```python
from build123d import *

# Parameters (mm, degrees)
SKETCH1_W           = 76.2
SKETCH1_H           = 25.4
SKETCH1_W_2         = 69.85
SKETCH1_H_2         = 19.05
BOSS_EXTRUDE1_DEPTH = 254
SKETCH2_R           = 3.3782
CUT_EXTRUDE1_DEPTH  = 26.4
SKETCH3_R           = 3
CUT_EXTRUDE2_DEPTH  = 26.4


with BuildPart() as part:
    # Sketch1 → Boss-Extrude1 (new body)
    with BuildSketch(Plane(origin=(0, 0, 0), x_dir=(1, 0, 0), z_dir=(0, 1, 0))):
        with Locations((38.1, 12.7)):
            Rectangle(SKETCH1_W, SKETCH1_H)
        with Locations((38.1, 12.7)):
            Rectangle(SKETCH1_W_2, SKETCH1_H_2, mode=Mode.SUBTRACT)
    extrude(amount=BOSS_EXTRUDE1_DEPTH)

    # Sketch2 → Cut-Extrude1 (cut, through all)
    with BuildSketch(Plane(origin=(0, 0, -25.4), x_dir=(-1, 0, 0), z_dir=(0, 0, -1))):
        with Locations((-60.325, 15.875)):
            Circle(SKETCH2_R)
        with Locations((-15.875, 15.875)):
            Circle(SKETCH2_R)
        with Locations((-15.875, 60.325)):
            Circle(SKETCH2_R)
        with Locations((-60.325, 60.325)):
            Circle(SKETCH2_R)
    extrude(amount=-CUT_EXTRUDE1_DEPTH, mode=Mode.SUBTRACT)

    # Sketch3 → Cut-Extrude2 (cut, through all)
    with BuildSketch(Plane(origin=(0, 0, -25.4), x_dir=(-1, 0, 0), z_dir=(0, 0, -1))):
        with Locations((-65.347432125, 185.7375)):
            Circle(SKETCH3_R)
        with Locations((-65.347432125, 233.3625)):
            Circle(SKETCH3_R)
    extrude(amount=-CUT_EXTRUDE2_DEPTH, mode=Mode.SUBTRACT)


solid = part.part
```
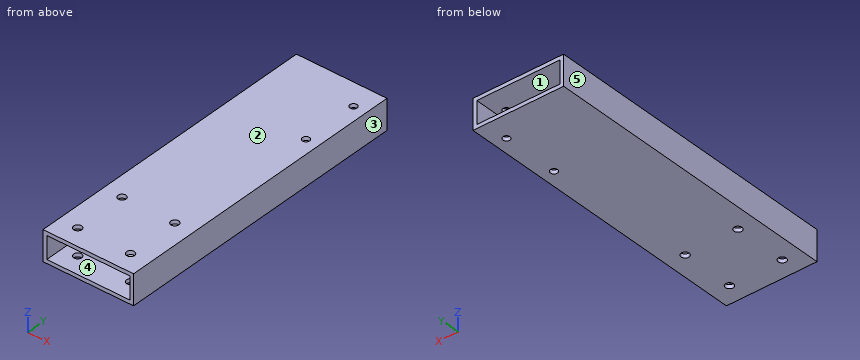
Could you check a few things on this model? Use its own coordinates, in mm. Face numbers are marked on the shaded views. A direction names the side the tool comes from. Coordinates: 2 decimals unless noted, no trailing zeros. Write each loop counter-clockwise with the first axis right and the second up, starting at its lowest first coordinate (ties: lowest second). Pieces come first, ordered by that corner, then holes. Notation, with made-up numbers: (58, 31) -> (94, 31) arc R23 cw to (94, 65) -> close; hole circle Ø3 at (-27, -3.75). An arc over 180 degrees is marked (long way). Return JSON: item names as keys, results as strings.
(1) I'm going to push a flat-ended pin straight in: pin 1 (4 mm diameter, centred on x = 15.875, y = 15.875, fed in from -Z). Where does the tip first touch, or does it pass through?
Numbers:
{"pin 1": "passes through"}
(2) Imagine slicing it at A-A, the plane x = 41. Please give me the cut outline in (y, z) (3 decimals), then the cut area to 3 significant figures.
Numbers:
{"outline": "(0, -25.4) -> (254, -25.4) -> (254, -22.225) -> (0, -22.225) -> close; (0, -3.175) -> (254, -3.175) -> (254, 0) -> (0, 0) -> close", "area": "1,610 mm2"}
(3) Imagine slicing it at B-B, the plane z = -12.75. Please give me the cut outline in (x, y) (3 decimals).
Numbers:
{"outline": "(0, 0) -> (3.175, 0) -> (3.175, 254) -> (0, 254) -> close; (73.025, 0) -> (76.2, 0) -> (76.2, 254) -> (73.025, 254) -> close"}
(4) Which directions (+Z, -Z, +X, -X, +Y, -Y) give clear straight access to the entire face, cutting with the end or side of a thin tool? Please do the marked faces 4 and 5.
Numbers:
{"face 4": "+Y, -Y", "face 5": "+Z, -Z, -X, +Y, -Y"}
(5) I need wall thicknesses on L1, parallel to X at y = 105, z = -8.5 (3 decimals); L2, parallel to Z at x = 30.5, y = 232.5 (3 decimals). Which ranges of each line are inside material? Lowest first, please.
Numbers:
{"L1": "x = 0 to 3.175, 73.025 to 76.2", "L2": "z = -25.4 to -22.225, -3.175 to 0"}
(6) Imagine slicing it at C-C, the plane y = 67. Please give me the cut outline in (x, z) (3 decimals).
Numbers:
{"outline": "(0, -25.4) -> (76.2, -25.4) -> (76.2, 0) -> (0, 0) -> close; hole (3.175, -22.225) -> (73.025, -22.225) -> (73.025, -3.175) -> (3.175, -3.175) -> close"}
(7) We'd pull the mould along X, two halves only. Please class the marked faces 1, 2 and 3: +X half, -X half, draft (parallel to the pull), parting line (faces both ways), or undercut.
Numbers:
{"face 1": "undercut", "face 2": "draft", "face 3": "+X half"}
